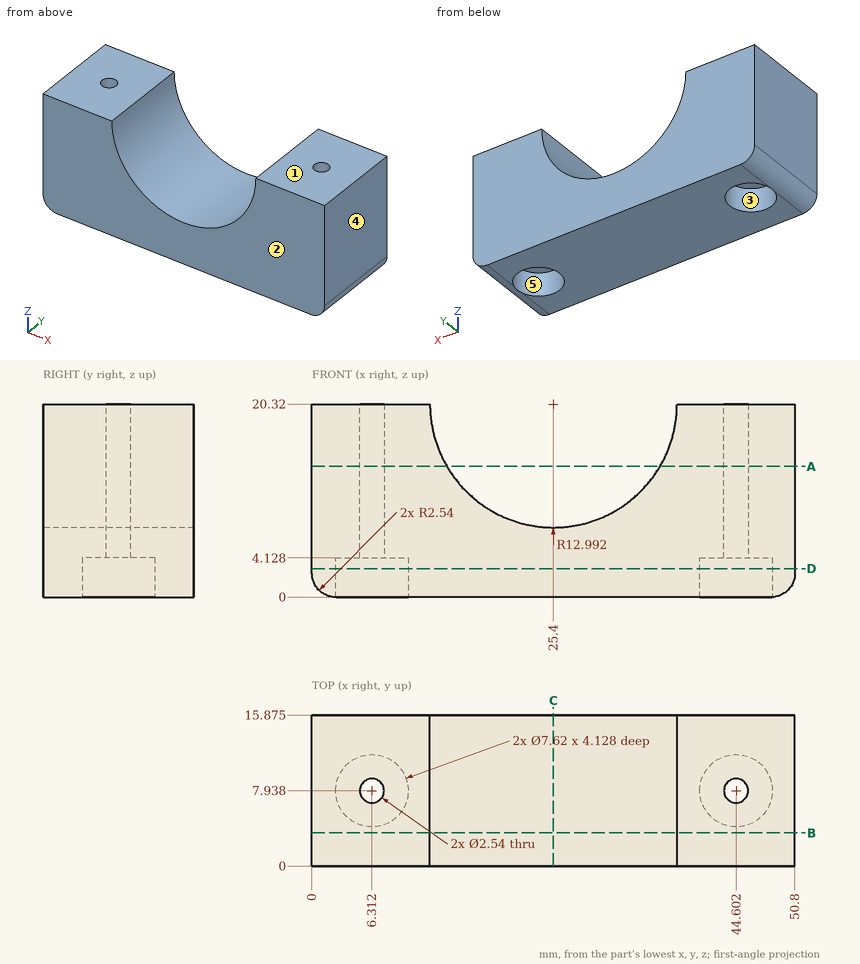
Could you check a few things on this drawing? It's one solid part, dimensions in mm from its lowest x, y, z. A direction names the side the tool comes from. Give positions to 0.01 mm unless a question says otherwise; leave off trailing zeros. Write each loop counter-clockwise with the first axis right and the second up, starting at its lowest first coordinate (ties: lowest second). Pieces come first, ordered by that corner, then holes.
(1) Thinking about a two-plate mould opening in Y: for the marked faces 1, 2 and 3, which applies, pulls with the +Y half, pulls with the -Y half, needs draft (parallel to the pull), parting line crosses it, or undercut?
Output values:
face 1: needs draft
face 2: pulls with the -Y half
face 3: undercut
(2) Imagine slicing it at A-A, the plane z = 13.75. Write out the boundary of the cut face in (x, y) (1 decimal).
Output values:
outline: (0, 0) - (14.2, 0) - (14.2, 15.9) - (0, 15.9) - close; (36.6, 0) - (50.8, 0) - (50.8, 15.9) - (36.6, 15.9) - close; hole circle Ø2.5 at (6.3, 7.9); hole circle Ø2.5 at (44.6, 7.9)
(3) Imagine slicing it at D-D, the plane z = 3. Write out the boundary of the cut face in (x, y) (1 decimal).
Output values:
outline: (0, 0) - (50.8, 0) - (50.8, 15.9) - (0, 15.9) - close; hole circle Ø7.6 at (6.3, 7.9); hole circle Ø7.6 at (44.6, 7.9)
(4) Imagine slicing it at B-B, the plane y = 3.5. Write out the boundary of the cut face in (x, z) (1 decimal).
Output values:
outline: (0, 2.5) arc R2.5 ccw to (2.5, 0) - (48.3, 0) arc R2.5 ccw to (50.8, 2.5) - (50.8, 20.3) - (38.4, 20.3) arc R13 cw to (12.4, 20.3) - (0, 20.3) - close
(5) If I drill on L1, parallel to X at y = 7.5, z = 18.5 (1 decimal); L2, parallel to Z at x = 8, y = 8.25; L3, parallel to X at y = 8, z = 12 (1 decimal), over which ranges is the centre line in solid material (lowest first)?
Output values:
L1: x = 0 to 5.1, 7.5 to 12.5, 38.3 to 43.4, 45.8 to 50.8
L2: z = 4.13 to 20.32
L3: x = 0 to 5, 7.6 to 15.4, 35.4 to 43.3, 45.9 to 50.8
(6) Imagine slicing it at C-C, the plane x = 25.4. Write out the boundary of the cut face in (y, z) (1 decimal), and give its area (3 significant figures).
Output values:
outline: (0, 0) - (15.9, 0) - (15.9, 7.3) - (0, 7.3) - close
area: 116 mm2
(7) Will these pins go through, and if not, where does the flat tip stop? pin 1 (7 mm diameter, centred on x = 44.6, y = 7.94, fed in from +Z); pin 2 (2.5 mm diameter, centred on x = 4.5, y = 6.5, fed in from -Z).
Output values:
pin 1: stops at z = 20.32
pin 2: stops at z = 4.13
(8) On a 3-axis mill with a long thin cutter (end or side, diameter ignored), from which of +Z, -Z, +X, -X, +Y, -Y can I reach the whole of each face in a straight line? I mean the marked faces 4 and 5. Say none if no direction works.
Output values:
face 4: +Z, -Z, +X, +Y, -Y
face 5: -Z
